The model under review builds one solid part; all positions refer to its coordinate system, in mm. A direction names the side the tool comes from. Round coordinates to 2 decimals unless told otherwise and drop trailing zeros. Order: outer loops, then holes, each group sorted by start corner. A loop starts at its lowest first (then second) coordinate and runs counter-clockwise, first axis right, second up. Notation, with made-up numbers: M 35.25,53 L 52.25,53 A23 cw 52.25,92 Z; hole C 28,76 d3. An arc over 180 degrees is marked long. One line per item, written item: value. Start each with the question number.
from build123d import *

# Parameters (mm, degrees)
SALIENTE_EXTRUIR1_DEPTH = 3


with BuildPart() as part:
    # Croquis1 → Saliente-Extruir1 (new body)
    with BuildSketch(Plane(origin=(0, 0, 0), x_dir=(1, 0, 0), z_dir=(0, 1, 0))):
        with BuildLine():
            Line((34.51, 4), (34.51, 0))
            Line((34.51, 0), (37.51, 0))
            Line((37.51, 0), (37.51, -2))
            Line((37.51, -2), (46.251262658, -2))
            ThreePointArc((46.251262658, -2), (59.584248365, -7.522703507), (65.106951872, -20.855689213))
            ThreePointArc((65.106951872, -20.855689213), (65.106606786, -20.969766147), (65.105571541, -21.083838906))
            Line((65.105571541, -21.083838906), (65, -38.533358743))
            Line((65, -38.533358743), (65, -86))
            Line((65, -86), (68, -86))
            Line((68, -86), (68, -96))
            Line((68, -96), (65, -96))
            Line((65, -96), (65, -117.736951872))
            Line((65, -117.736951872), (65, -188.736951872))
            Line((65, -188.736951872), (67, -188.736951872))
            Line((67, -188.736951872), (67, -191.736951872))
            Line((67, -191.736951872), (75, -191.736951872))
            Line((75, -191.736951872), (75, -188.736951872))
            Line((75, -188.736951872), (77, -188.736951872))
            Line((77, -188.736951872), (77, -96))
            Line((77, -96), (74, -96))
            Line((74, -96), (74, -86))
            Line((74, -86), (77, -86))
            Line((77, -86), (77, -64.74))
            Line((77, -64.74), (77, -38.533358743))
            Line((77, -38.533358743), (77, -23.422537226))
            Line((77, -23.422537226), (77, -18.2888412))
            ThreePointArc((77, -18.2888412), (67.142309691, 1.851968321), (46.251262658, 10))
            Line((46.251262658, 10), (37.51, 10))
            Line((37.51, 10), (37.51, 8))
            Line((37.51, 8), (34.51, 8))
            Line((34.51, 8), (34.51, 4))
        make_face()
        Polygon((67.200961894, -61.159872981), (69.799038106, -59.659872981), (74.799038106, -68.320127019), (72.200961894, -69.820127019), align=None, mode=Mode.SUBTRACT)
    extrude(amount=SALIENTE_EXTRUIR1_DEPTH)


solid = part.part
Item 1: The part is to be moulded in two halves that separate along Z. For faces 1 (the flat face through (72.264, 1.479, 63.929)), 2 (the cylindrical face through (67.38, 1.48, -1.63)), 3 (the flat face through (67, 3, 83)), say which applies: pulls with the +Z half, pulls with the -Z half, needs draft (parallel to the pull), parting line crosses it, or undercut.
Item 2: Machinability: for faces 4 (the flat face through (69.736, 1.479, 65.551)), 5 (the flat face through (67, 0, 83)), which of the approach directions +Z, -Z, +X, -X, +Y, -Y give a long, thin tool a straight path to every point of the face, cutting with its end or side? Answer none if there is none.
Item 3: Consider section C-C, the plane z = 148. Give the boundary of the cut face in (x, y).
Item 4: Consider section B-B, the plane x = 43.5. Give the boundary of the cut face in (y, z), then the cut area to 3 significant figures.
Item 5: Clearance check with flat-ended pins moving along their axes: P1, Ø1, axis at y = 1.5, z = -9.5, coming from the -X side; P2, Ø1, axis at x = 66, y = 2, coming from the +Z side; P3, Ø0.9, axis at y = 1.5, z = 71, coming from the -X side. State where each tip first meets the part, or that it passes through.
Item 6: Wall thickness on L1, parallel to X at y = 0.85, z = 162.5; L2, parallel to Z at x = 72.5, y = 2.7; L3, parallel to Z at x = 44.5, y = 1.2: over which ranges is each line inside the solid? List them lowest first.
Computed:
1. face 1: undercut
1. face 2: pulls with the -Z half
1. face 3: needs draft
2. face 4: +Y, -Y
2. face 5: +Z, -Z, +X, -X, -Y
3. outline: M 65,0 L 77,0 L 77,3 L 65,3 Z
4. outline: M 0,-10 L 3,-10 L 3,2 L 0,2 Z
4. area: 36.0 mm^2
5. P1: stops at x = 37.51
5. P2: stops at z = 188.74
5. P3: stops at x = 65
6. L1: x = 65 to 77
6. L2: z = 4.64 to 64.34, 69.65 to 191.74
6. L3: z = -10 to 2
